```python
from build123d import *

# Parameters (mm, degrees)
BOX002_W          = 6.25
BOX002_H          = 6
BOX002_DEPTH      = 10
BOX001_W          = 6.25
BOX001_H          = 6
BOX001_DEPTH      = 10
CYLINDER001_R     = 2.8
CYLINDER001_DEPTH = 10
CYLINDER_R        = 2.8
CYLINDER_DEPTH    = 10
BOX_W             = 47
BOX_H             = 51
BOX_DEPTH         = 5
FILLET_R          = 1
FILLET001_R       = 1
FILLET002_R       = 1


with BuildPart() as cube002:
    # Box002 → Box002 (new body)
    with BuildSketch(Plane(origin=(40.75, 30.25, -2), x_dir=(1, 0, 0), z_dir=(0, 0, 1))):
        with Locations((3.125, 3)):
            Rectangle(BOX002_W, BOX002_H)
    extrude(amount=BOX002_DEPTH)


with BuildPart() as fusion:
    # Box001 → Box001 (new body)
    with BuildSketch(Plane(origin=(0, 30.25, -2), x_dir=(1, 0, 0), z_dir=(0, 0, 1))):
        with Locations((3.125, 3)):
            Rectangle(BOX001_W, BOX001_H)
    extrude(amount=BOX001_DEPTH)

    # Fusion: union Cube002
    add(cube002.part)


with BuildPart() as cylinder001:
    # Cylinder001 → Cylinder001 (new body)
    with BuildSketch(Plane(origin=(41.9, 6.9, -2), x_dir=(1, 0, 0), z_dir=(0, 0, 1))):
        Circle(CYLINDER001_R)
    extrude(amount=CYLINDER001_DEPTH)


with BuildPart() as cylinder:
    # Cylinder → Cylinder (new body)
    with BuildSketch(Plane(origin=(5.1, 42.6, -2), x_dir=(1, 0, 0), z_dir=(0, 0, 1))):
        Circle(CYLINDER_R)
    extrude(amount=CYLINDER_DEPTH)


with BuildPart() as fillet002:
    # Box → Box (new body)
    with BuildSketch(Plane.XY):
        with Locations((23.5, 25.5)):
            Rectangle(BOX_W, BOX_H)
    extrude(amount=BOX_DEPTH)

    # Cut: cut Cylinder
    add(cylinder.part, mode=Mode.SUBTRACT)

    # Cut001: cut Cylinder001
    add(cylinder001.part, mode=Mode.SUBTRACT)

    # Cut002: cut Fusion
    add(fusion.part, mode=Mode.SUBTRACT)

    # Fillet
    fillet_edges = [fillet002.edges().sort_by_distance(p)[0] for p in [
        (0, 0, 2.5),
        (47, 0, 2.5),
        (0, 51, 2.5),
        (47, 51, 2.5),
    ]]
    fillet(fillet_edges, radius=FILLET_R)

    # Fillet001
    fillet001_edges = [fillet002.edges().sort_by_distance(p)[0] for p in [
        (0, 30.25, 2.5),
        (0, 36.25, 2.5),
        (47, 30.25, 2.5),
        (47, 36.25, 2.5),
    ]]
    fillet(fillet001_edges, radius=FILLET001_R)

    # Fillet002
    fillet002_edges = [fillet002.edges().sort_by_distance(p)[0] for p in [
        (6.25, 30.25, 2.5),
        (6.25, 36.25, 2.5),
        (40.75, 30.25, 2.5),
        (40.75, 36.25, 2.5),
    ]]
    fillet(fillet002_edges, radius=FILLET002_R)


solid = fillet002.part
```
Part model, mm, in its own coordinate system. A direction names the side the tool comes from. Give positions to 0.01 mm unless a question says otherwise; leave off trailing zeros. Write each loop counter-clockwise with the first axis right and the second up, starting at its lowest first coordinate (ties: lowest second). Pieces come first, ordered by that corner, then holes. Notation, with made-up numbers: (66, -30.5) -> (103, -30.5) arc R17 ccw to (103, -19.5) -> close; hole circle Ø11 at (53, -19.75). An arc over 180 degrees is marked (long way). Put each result on its own line as item: value. Start each with the question number.
Item 1: Which spindle directions (+Z, -Z, +X, -X, +Y, -Y) get a long thin tool onto all of the face, cutting with end or side? Do faces 1 (the face through (3, 30.25, 2)), 2 (the face through (47, 44, 2)), 3 (the face through (44, 30.25, 2)). Say none if no direction does.
Item 2: Cut at A-A (y = 6.9). List the corners of the cut face in (x, z), then the cut area to 3 significant figures.
Item 3: Cut at B-B (z = 0.9). List the corners of the cut face in (x, y).
Item 4: Cut at C-C (x = 43.5). List the corners of the cut face in (y, z).
Item 5: Wall check: L1, parallel to Y at x = 5.1, z = 3.5; L2, parallel to Y at x = 41.9, z = 1.1; L3, parallel to X at y = 6.9, z = 3.9. Give the ranges that are in metal, low to high. Write a range as [from, to].
Item 6: Pull direction X, two halves, no side cores. Call faces 4 (the face through (39.1, 7, 2.5)), 5 (the face through (6.392, 40.116, 2.465)), 6 (the face through (40.75, 33, 2)), 7 (the face through (0, 44, 2)): pulls with the +X half, pulls with the -X half, needs draft (parallel to the pull), parting line crosses it, or undercut.
Item 7: Pin check, flat tips, straight feed: pin 1 Ø1.2 at (y, z) = (34, 2.5) entering from +X; pin 2 Ø3 at (y, z) = (32.5, 3) entering from -X. Stop position of each tip, or through.
Answer list:
1. face 1: +Z, -Z, -X
1. face 2: +Z, -Z, +X, +Y, -Y
1. face 3: +Z, -Z, +X
2. outline: (0, 0) -> (39.1, 0) -> (39.1, 5) -> (0, 5) -> close; (44.7, 0) -> (47, 0) -> (47, 5) -> (44.7, 5) -> close
2. area: 207 mm2
3. outline: (0, 1) arc R1 ccw to (1, 0) -> (46, 0) arc R1 ccw to (47, 1) -> (47, 29.25) arc R1 ccw to (46, 30.25) -> (41.75, 30.25) arc R1 cw to (40.75, 31.25) -> (40.75, 35.25) arc R1 cw to (41.75, 36.25) -> (46, 36.25) arc R1 ccw to (47, 37.25) -> (47, 50) arc R1 ccw to (46, 51) -> (1, 51) arc R1 ccw to (0, 50) -> (0, 37.25) arc R1 ccw to (1, 36.25) -> (5.25, 36.25) arc R1 cw to (6.25, 35.25) -> (6.25, 31.25) arc R1 cw to (5.25, 30.25) -> (1, 30.25) arc R1 ccw to (0, 29.25) -> close; hole circle Ø5.6 at (5.1, 42.6); hole circle Ø5.6 at (41.9, 6.9)
4. outline: (0, 0) -> (4.6, 0) -> (4.6, 5) -> (0, 5) -> close; (9.2, 0) -> (30.25, 0) -> (30.25, 5) -> (9.2, 5) -> close; (36.25, 0) -> (51, 0) -> (51, 5) -> (36.25, 5) -> close
5. L1: y = [0, 30.25], [36.25, 39.8], [45.4, 51]
5. L2: y = [0, 4.1], [9.7, 30.25], [36.25, 51]
5. L3: x = [0, 39.1], [44.7, 47]
6. face 4: undercut
6. face 5: undercut
6. face 6: pulls with the +X half
6. face 7: pulls with the -X half
7. pin 1: stops at x = 40.75
7. pin 2: stops at x = 6.22
